Geometry: final body of the model. Coordinates: model frame, mm. A direction names the side the tool comes from. Coordinates: 2 decimals unless noted, no trailing zeros. Order: outer loops, then holes, each group sorted by start corner. A loop starts at its lowest first (then second) coordinate and runs counter-clockwise, first axis right, second up. Notation, with made-up numbers: M 55.25,34.5 L 74.25,34.5 A19 ccw 74.25,42.5 Z; hole C 72.5,-37 d4. An arc over 180 degrees is marked long. One line per question, with ' | ' between items.
from build123d import *

# Parameters (mm, degrees)
SKETCH1_R               = 15.1
SKETCH1_R_2             = 10.1
BOSS_EXTRUDE1_DEPTH     = 7
CUT_EXTRUDE3_DEPTH      = 22
CUT_EXTRUDE3_DEPTH_BACK = 24
SKETCH4_R               = 23.353820798
SKETCH4_R_2             = 11.1
CUT_EXTRUDE4_DEPTH      = 1
SKETCH6_R               = 15.1
SKETCH6_R_2             = 10.1
BOSS_EXTRUDE2_DEPTH     = 0.8


with BuildPart() as part:
    # Sketch1 → Boss-Extrude1 (new body)
    with BuildSketch(Plane(origin=(0, 0, 0), x_dir=(1, 0, 0), z_dir=(0, 1, 0))):
        with Locations(Location((0, 0, 0), (0, 0, 270))):
            Circle(SKETCH1_R)
        with Locations(Location((0, 0, 0), (0, 0, 270))):
            Circle(SKETCH1_R_2, mode=Mode.SUBTRACT)
    extrude(amount=BOSS_EXTRUDE1_DEPTH)

    # Sketch2 → Cut-Extrude3 (cut, two sides: drawn at the far end of the back side and taken through both)
    with BuildSketch(Plane(origin=(0, 0, 0), x_dir=(0, 0, -1), z_dir=(1, 0, 0)).offset(-CUT_EXTRUDE3_DEPTH_BACK)):
        with BuildLine():
            Line((0, 5.901951984), (0, 4.401951984))
            Line((0, 4.401951984), (0, 3.5))
            Line((0, 3.5), (0, 2.901951984))
            ThreePointArc((0, 2.901951984), (1.060660172, 3.341291812), (1.5, 4.401951984))
            ThreePointArc((1.5, 4.401951984), (1.060660172, 5.462612156), (0, 5.901951984))
        make_face()
        with BuildLine():
            Line((0, 3.5), (0, 4.401951984))
            Line((0, 4.401951984), (0, 5.901951984))
            ThreePointArc((0, 5.901951984), (-1.5, 4.401951984), (0, 2.901951984))
            Line((0, 2.901951984), (0, 3.5))
        make_face()
    extrude(amount=CUT_EXTRUDE3_DEPTH + CUT_EXTRUDE3_DEPTH_BACK, mode=Mode.SUBTRACT)

    # Sketch4 → Cut-Extrude4 (cut)
    with BuildSketch(Plane.XZ):
        Circle(SKETCH4_R)
        with Locations(Location((0, 0, 0), (0, 0, 270))):
            Circle(SKETCH4_R_2, mode=Mode.SUBTRACT)
    extrude(amount=-CUT_EXTRUDE4_DEPTH, mode=Mode.SUBTRACT)

    # Sketch6 → Boss-Extrude2 (add)
    with BuildSketch(Plane(origin=(0, 7, 0), x_dir=(1, 0, 0), z_dir=(0, 1, 0))):
        with Locations(Location((0, 0, 0), (0, 0, 90))):
            Circle(SKETCH6_R)
        with Locations(Location((0, 0, 0), (0, 0, 270))):
            Circle(SKETCH6_R_2, mode=Mode.SUBTRACT)
    extrude(amount=BOSS_EXTRUDE2_DEPTH)


solid = part.part
1. Section D-D, the plane x = 13.5. Output: boundary loops of the cut face in (y, z), and give its area (3 significant figures).
Response values:
outline: M 1,-6.76 L 7.8,-6.76 L 7.8,6.76 L 1,6.76 Z; hole C 4.4,0 d3 | area: 84.9 mm^2
2. Pin query (flat end, axial travel): P1, Ø1, axis at x = -2.5, y = 1.5, coming from the -Z side; P2, Ø1.5, axis at y = 2.5, z = -5.5, coming from the +X side; P3, Ø2, axis at y = 3, z = 9, coming from the -X side; P4, Ø9, axis at x = 0.5, z = 7.5, coming from the -Y side. Return the tip coordinate at first contact, or that it passes through.
Response values:
P1: stops at z = -14.97 | P2: stops at x = 14.33 | P3: stops at x = -12.81 | P4: stops at y = 0
3. Access query for faces 1 (the face through (10, 7.8, -3)), 2 (the face through (-8, 1, 8)). Directions: +Z, -Z, +X, -X, +Y, -Y. A direction counts if a zero-diameter tool reaches every point of the face in a straight line with its end or side. Return the directions, or none.
Response values:
face 1: +Z, -Z, +X, -X, +Y | face 2: -Y
4. Section A-A, the plane x = 0. Output: boundary loops of the cut face in (y, z), and give its area (3 significant figures).
Response values:
outline: M 0,-11.1 L 1,-11.1 L 1,-15.1 L 7.8,-15.1 L 7.8,-10.1 L 0,-10.1 Z; M 0,10.1 L 7.8,10.1 L 7.8,15.1 L 1,15.1 L 1,11.1 L 0,11.1 Z | area: 70.0 mm^2
5. Section C-C, the plane z = -8.5. Output: boundary loops of the cut face in (x, y).
Response values:
outline: M -12.48,1 L -7.14,1 L -7.14,0 L -5.46,0 L -5.46,7.8 L -12.48,7.8 Z; M 5.46,0 L 7.14,0 L 7.14,1 L 12.48,1 L 12.48,7.8 L 5.46,7.8 Z
6. Material intervals for line 1 (X direction, y = 7.25, z = 0); line 2 (Y direction, x = 0.5, z = 12); line 3 (X direction, y = 6.5, z = -3.5), sorted ascending. Write a range as [from, to].
Response values:
line 1: x = [-15.1, -10.1], [10.1, 15.1] | line 2: y = [1, 7.8] | line 3: x = [-14.69, -9.47], [9.47, 14.69]
7. Section B-B, the plane y = 3.75. Output: boundary loops of the cut face in (x, z), and give its area (3 significant figures).
Response values:
outline: M -15.04,-1.35 A15.1 ccw 15.04,-1.35 L 10.01,-1.35 A10.1 cw -10.01,-1.35 Z; M -15.04,1.35 L -10.01,1.35 A10.1 cw 10.01,1.35 L 15.04,1.35 A15.1 ccw Z | area: 369 mm^2
